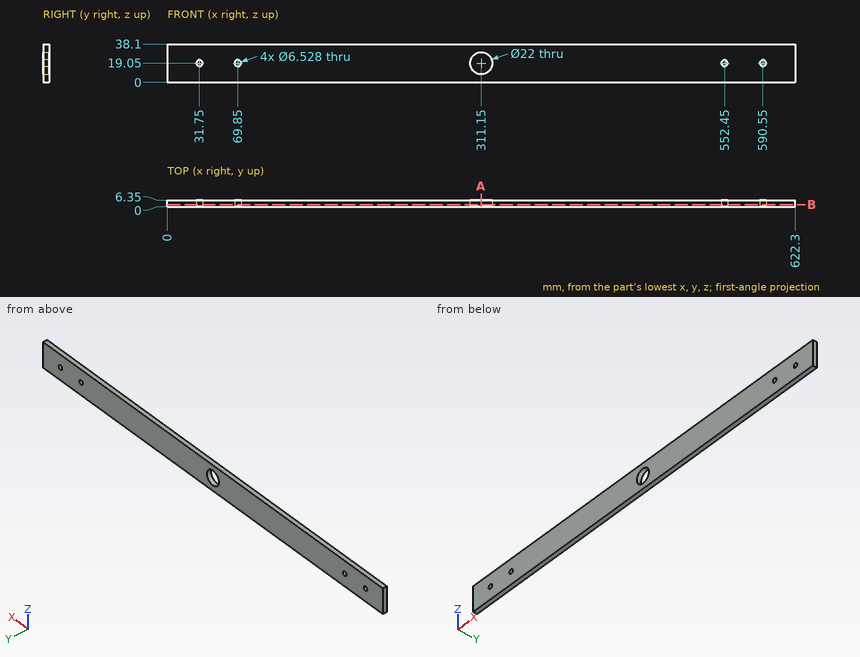
Design review of the part shown in the three views and the two pictorial views. Dimensions are in mm from the part's minimum x, y and z. Round coordinates to 2 decimals unless told otherwise and drop trailing zeros. Write each loop counter-clockwise with the first axis right and the second up, starting at its lowest first coordinate (ties: lowest second). Pieces come first, ordered by that corner, then holes.
Item 1: Wall thickness on L1, parallel to Z at x = 69.85, y = 3; L2, parallel to X at y = 5.5, z = 22 (1 decimal); L3, parallel to X at y = 5.5, z = 9.5: over which ranges is each line inside the solid? List them lowest first.
Item 2: Consider section B-B on y = 2.25. Give the boundary of the cut face in (x, z).
Item 3: Consider section A-A on x = 311.15. Give the boundary of the cut face in (y, z), and give its area (3 significant figures).
Check values:
1. L1: z = 0 to 15.79, 22.31 to 38.1
1. L2: x = 0 to 30.4, 33.1 to 68.5, 71.2 to 300.6, 321.7 to 551.1, 553.8 to 589.2, 591.9 to 622.3
1. L3: x = 0 to 305.69, 316.61 to 622.3
2. outline: (0, 0) - (622.3, 0) - (622.3, 38.1) - (0, 38.1) - close; hole circle Ø6.53 at (31.75, 19.05); hole circle Ø6.53 at (69.85, 19.05); hole circle Ø22 at (311.15, 19.05); hole circle Ø6.53 at (552.45, 19.05); hole circle Ø6.53 at (590.55, 19.05)
3. outline: (0, 0) - (6.35, 0) - (6.35, 8.05) - (0, 8.05) - close; (0, 30.05) - (6.35, 30.05) - (6.35, 38.1) - (0, 38.1) - close
3. area: 102 mm2
